from build123d import *

# Parameters (mm, degrees)
BOSS_EXTRUDE1_DEPTH = 1.5
BOSS_EXTRUDE2_START = -10
BOSS_EXTRUDE2_DEPTH = 10
BOSS_EXTRUDE3_START = -50
BOSS_EXTRUDE3_DEPTH = 10
FILLET1_R           = 2


with BuildPart() as part:
    # Sketch1 → Boss-Extrude1 (new body)
    with BuildSketch(Plane(origin=(0, 0, 0), x_dir=(1, 0, 0), z_dir=(0, 1, 0))):
        with BuildLine():
            Line((2.414213562, 0), (69.385786438, 0))
            ThreePointArc((69.385786438, 0), (69.794034728, 0.211324865), (69.857190958, 0.666666667))
            ThreePointArc((69.857190958, 0.666666667), (70.092893219, 1.707106781), (71.133333333, 1.942809042))
            ThreePointArc((71.133333333, 1.942809042), (71.588675135, 2.005965272), (71.8, 2.414213562))
            Line((71.8, 2.414213562), (71.8, 34.385786438))
            ThreePointArc((71.8, 34.385786438), (71.588675135, 34.794034728), (71.133333333, 34.857190958))
            ThreePointArc((71.133333333, 34.857190958), (70.092893219, 35.092893219), (69.857190958, 36.133333333))
            ThreePointArc((69.857190958, 36.133333333), (69.794034728, 36.588675135), (69.385786438, 36.8))
            Line((69.385786438, 36.8), (2.414213562, 36.8))
            ThreePointArc((2.414213562, 36.8), (2.005965272, 36.588675135), (1.942809042, 36.133333333))
            ThreePointArc((1.942809042, 36.133333333), (1.707106781, 35.092893219), (0.666666667, 34.857190958))
            ThreePointArc((0.666666667, 34.857190958), (0.211324865, 34.794034728), (0, 34.385786438))
            Line((0, 34.385786438), (0, 2.414213562))
            ThreePointArc((0, 2.414213562), (0.211324865, 2.005965272), (0.666666667, 1.942809042))
            ThreePointArc((0.666666667, 1.942809042), (1.707106781, 1.707106781), (1.942809042, 0.666666667))
            ThreePointArc((1.942809042, 0.666666667), (2.005965272, 0.211324865), (2.414213562, 0))
        make_face()
    extrude(amount=BOSS_EXTRUDE1_DEPTH)

    # Sketch3 → Boss-Extrude2 (add)
    with BuildSketch(Plane.ZY.offset(BOSS_EXTRUDE2_START)):
        with BuildLine():
            Line((-12.374014603, 0), (-24.425985397, 0))
            ThreePointArc((-24.425985397, 0), (-28.666594565, -4.90005043), (-29.500762028, -11.326357689))
            add(Edge.make_bspline(
                [(-29.500762028, -11.326357689), (-28.897266876, -13.751803061), (-29.879831091, -16.043728976)],
                knots=[0, 0, 0, 1, 1, 1], degree=2))
            ThreePointArc((-29.879831091, -16.043728976), (-29.693870441, -16.6908382), (-29.032229169, -16.566088301))
            add(Edge.make_bspline(
                [(-27.599358013, -10.46659824), (-26.907734986, -13.817809078), (-29.032229169, -16.566088301)],
                knots=[0, 0, 0, 1, 1, 1], degree=2))
            ThreePointArc((-27.599358013, -10.46659824), (-18.4, -0.25), (-9.200641987, -10.46659824))
            add(Edge.make_bspline(
                [(-9.200641987, -10.46659824), (-9.892265014, -13.817809078), (-7.767770831, -16.566088301)],
                knots=[0, 0, 0, 1, 1, 1], degree=2))
            ThreePointArc((-7.767770831, -16.566088301), (-7.106129559, -16.6908382), (-6.920168909, -16.043728976))
            add(Edge.make_bspline(
                [(-7.299237972, -11.326357689), (-7.902733124, -13.751803061), (-6.920168909, -16.043728976)],
                knots=[0, 0, 0, 1, 1, 1], degree=2))
            ThreePointArc((-7.299237972, -11.326357689), (-8.133405435, -4.90005043), (-12.374014603, 0))
        make_face()
    extrude(amount=-BOSS_EXTRUDE2_DEPTH)

    # Sketch3_3 → Boss-Extrude3 (add)
    with BuildSketch(Plane.ZY.offset(BOSS_EXTRUDE3_START)):
        with BuildLine():
            Line((-12.374014603, 0), (-24.425985397, 0))
            ThreePointArc((-24.425985397, 0), (-28.666594565, -4.90005043), (-29.500762028, -11.326357689))
            add(Edge.make_bspline(
                [(-29.500762028, -11.326357689), (-28.897266876, -13.751803061), (-29.879831091, -16.043728976)],
                knots=[0, 0, 0, 1, 1, 1], degree=2))
            ThreePointArc((-29.879831091, -16.043728976), (-29.693870441, -16.6908382), (-29.032229169, -16.566088301))
            add(Edge.make_bspline(
                [(-27.599358013, -10.46659824), (-26.907734986, -13.817809078), (-29.032229169, -16.566088301)],
                knots=[0, 0, 0, 1, 1, 1], degree=2))
            ThreePointArc((-27.599358013, -10.46659824), (-18.4, -0.25), (-9.200641987, -10.46659824))
            add(Edge.make_bspline(
                [(-9.200641987, -10.46659824), (-9.892265014, -13.817809078), (-7.767770831, -16.566088301)],
                knots=[0, 0, 0, 1, 1, 1], degree=2))
            ThreePointArc((-7.767770831, -16.566088301), (-7.106129559, -16.6908382), (-6.920168909, -16.043728976))
            add(Edge.make_bspline(
                [(-7.299237972, -11.326357689), (-7.902733124, -13.751803061), (-6.920168909, -16.043728976)],
                knots=[0, 0, 0, 1, 1, 1], degree=2))
            ThreePointArc((-7.299237972, -11.326357689), (-8.133405435, -4.90005043), (-12.374014603, 0))
        make_face()
    extrude(amount=-BOSS_EXTRUDE3_DEPTH)

    # Fillet1
    fillet1_edges = [part.edges().sort_by_distance(p)[0] for p in [
        (15, 0, -24.425985397),
        (15, 0, -12.374014603),
        (55, 0, -24.425985397),
        (55, 0, -12.374014603),
    ]]
    fillet(fillet1_edges, radius=FILLET1_R)


solid = part.part
Design review of the part built by this model. Coordinates are the model's own, in mm. A direction names the side the tool comes from. Coordinates: 2 decimals unless noted, no trailing zeros. Write each loop counter-clockwise with the first axis right and the second up, starting at its lowest first coordinate (ties: lowest second). Pieces come first, ordered by that corner, then holes. Notation, with made-up numbers: (14.25, 74.25) -> (38.25, 74.25) arc R32 cw to (38.25, 113.25) -> close; hole circle Ø10 at (5, 60.5). An arc over 180 degrees is marked (long way). Write each question's results on one line, items separated by ' | '. Start each with the question number.
(1) Take a section at A-A on y = -8.75. Write out the cut boundary in (x, z), and give its area (3 significant figures).
(2) Tool access review of faces 1 (the face through (14.93, -0.253, -18.617)), 2 (the face through (54.93, -6.994, -29.367)), 3 (the face through (10, -0.3, -15.9)), 4 (the face through (20, -0.3, -15.9)): name each direction out of +Z, -Z, +X, -X, +Y, -Y from which nothing blocks a thin tool from reaching the whole face with its end or side.
(3) Take a section at B-B on z = -18.4. Write out the cut boundary in (x, y), and give its area (3 significant figures).
(4) Take a section at D-D on y = -2. Write out the cut boundary in (x, z), and give its area (3 significant figures).
(5) The part is to be moulded in two halves that separate along Z. For faces 5 (the face through (1.696, 0.74, -1.718)), 6 (the face through (60, -0.3, -15.9)), 7 (the face through (35, 1, 0)), say which applies: pulls with the +Z half, pulls with the -Z half, needs draft (parallel to the pull), parting line crosses it, or undercut.
(6) Clearance check with flat-ended pins moving along their axes: P1, Ø1, axis at x = 60, y = -14.5, coming from the +Z side; P2, Ø4, axis at y = -3.5, z = -26, coming from the +X side; P3, Ø4, axis at x = 51, y = -4, coming from the +Z side. State where each tip first meets the part, or that it passes through.
(7) Take a section at C-C on x = 33. Write out the cut boundary in (y, z).
(8) For line 1 along Z through (x, y) = (54.75, -9.5); line 2 along X through (y, z) = (-7.75, -28.5); line 3 along Y through (x, z) = (4.5, -31), list the stretches that pass through material, from the lowest coordinate up. Write a range as from..to.
Results found:
1) outline: (10, -29.62) -> (20, -29.62) -> (20, -27.62) -> (10, -27.62) -> close; (10, -9.18) -> (20, -9.18) -> (20, -7.18) -> (10, -7.18) -> close; (50, -29.62) -> (60, -29.62) -> (60, -27.62) -> (50, -27.62) -> close; (50, -9.18) -> (60, -9.18) -> (60, -7.18) -> (50, -7.18) -> close | area: 80.2 mm2
2) face 1: +X, -X | face 2: -Z, +X, -X | face 3: +Z, -Z, -X, -Y | face 4: +Z, -Z, -Y
3) outline: (0, 0) -> (10, 0) -> (10, -0.25) -> (20, -0.25) -> (20, 0) -> (50, 0) -> (50, -0.25) -> (60, -0.25) -> (60, 0) -> (71.8, 0) -> (71.8, 1.5) -> (0, 1.5) -> close | area: 113 mm2
4) outline: (10, -27.32) -> (20, -27.32) -> (20, -23.81) -> (10, -23.81) -> close; (10, -12.99) -> (20, -12.99) -> (20, -9.48) -> (10, -9.48) -> close; (50, -27.32) -> (60, -27.32) -> (60, -23.81) -> (50, -23.81) -> close; (50, -12.99) -> (60, -12.99) -> (60, -9.48) -> (50, -9.48) -> close | area: 140 mm2
5) face 5: undercut | face 6: needs draft | face 7: pulls with the +Z half
6) P1: stops at z = -7.28 | P2: stops at x = 60 | P3: stops at z = -7.71
7) outline: (0, -36.8) -> (1.5, -36.8) -> (1.5, 0) -> (0, 0) -> close
8) line 1: z = -29.65..-27.65, -9.15..-7.15 | line 2: x = 10..20, 50..60 | line 3: y = 0..1.5
